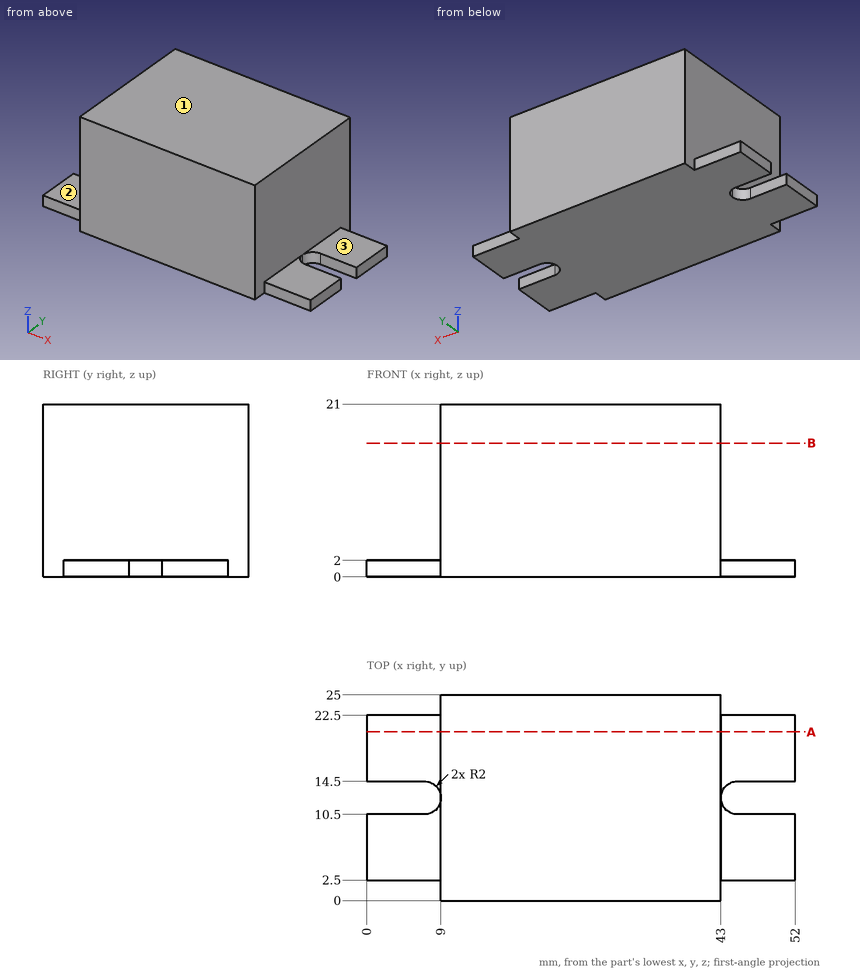
Part print with two shaded views. Sizes in mm from the minimum x, y, z corner. A direction names the side the tool comes from. Give positions to 0.01 mm unless a question says otherwise; leave off trailing zeros. Write each loop counter-clockwise with the first axis right and the second up, starting at its lowest first coordinate (ties: lowest second). Pieces come first, ordered by that corner, then holes.
1) Cut at B-B on z = 16.25. Write the cut outline in (x, y), then the cut area to 3 significant figures.
Resolved:
outline: (9, 0) - (43, 0) - (43, 25) - (9, 25) - close
area: 850 mm2
2) Pin check, flat tips, straight feed: pin 1 (7 mm diameter, centred on x = 49, y = 7, fed in from +Z); pin 2 (1 mm diameter, centred on x = 49.5, z = 1, fed in from +Y); pin 3 (1.6 mm diameter, centred on x = 2, z = 1, fed in from -Y). Stop position of each tip, or through.
Resolved:
pin 1: stops at z = 2
pin 2: stops at y = 22.5
pin 3: stops at y = 2.5
3) Which spindle directions (+Z, -Z, +X, -X, +Y, -Y) get a long thin tool onto all of the face, cutting with end or side? Do the marked faces 1, 2 and 3. Say none if no direction does.
Resolved:
face 1: +Z, +X, -X, +Y, -Y
face 2: +Z, -X, +Y, -Y
face 3: +Z, +X, +Y, -Y
4) Probe L1, parallel to X at y = 8.25, z = 15; L2, parallel to Z at x = 3.5, y = 7.5. List the from-to ranges inside material, lowest first.
Resolved:
L1: x = 9 to 43
L2: z = 0 to 2
5) Cut at A-A on y = 20.5. Write the cut outline in (x, z).
Resolved:
outline: (0, 0) - (52, 0) - (52, 2) - (43, 2) - (43, 21) - (9, 21) - (9, 2) - (0, 2) - close
